Part model, mm, in its own coordinate system. Face numbers are marked on the shaded views. A direction names the side the tool comes from. Coordinates: 2 decimals unless noted, no trailing zeros. Order: outer loops, then holes, each group sorted by start corner. A loop starts at its lowest first (then second) coordinate and runs counter-clockwise, first axis right, second up.
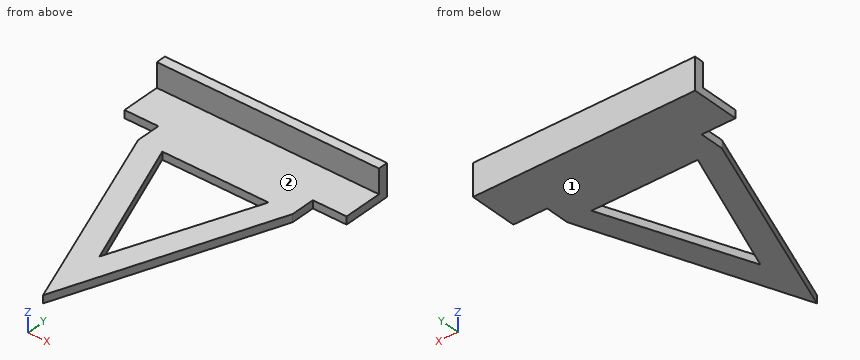
from build123d import *

# Parameters (mm, degrees)
F1_DEPTH = 1.6
F2_W     = 46
F2_H     = 2
F3_DEPTH = 5


with BuildPart() as f1:
    # F0 (on Top) → F1 (new body)
    with BuildSketch(Plane.XY):
        Polygon((23, 0), (0, 0), (-23, 0), (-23, -10), (-16, -10), (-16, -15), (0, -57.71), (16, -15), (16, -10), (23, -10), align=None)
        Polygon((0, -43.71), (-11, -15), (0, -15), (11, -15), align=None, mode=Mode.SUBTRACT)
    extrude(amount=F1_DEPTH)

    # F2 (on face) → F3 (join)
    with BuildSketch(Plane.XY.offset(1.6)):
        with Locations((0, -1)):
            Rectangle(F2_W, F2_H)
    extrude(amount=F3_DEPTH)


solid = f1.part
Q1. Cut at A-A on z = 0.75. Write the cut outline in (x, y).
Results list:
outline: (-23, -10) - (-16, -10) - (-16, -15) - (0, -57.71) - (16, -15) - (16, -10) - (23, -10) - (23, 0) - (-23, 0) - close; hole (-11, -15) - (0, -43.71) - (11, -15) - close
Q2. Pin check, flat tips, straight feed: pin 1 Ø1.3 at (y, z) = (-12.5, 1) entering from -X; pin 2 Ø6 at (x, y) = (-18, -22) entering from +Z; pin 3 Ø0.8 at (x, z) = (21, 1) entering from -Y; pin 4 Ø1.5 at (x, z) = (2, 4) entering from -Y. Stop position of each tip, or through.
Results list:
pin 1: stops at x = -16
pin 2: passes through
pin 3: stops at y = -10
pin 4: stops at y = -2
Q3. Wall check: line 1 along X through (y, z) = (-14.5, 1); line 2 along Y through (x, z) = (-17.5, 1); line 3 along Z through (x, y) = (-12, -17.5). Give the ranges that are in metal, low to high.
Results list:
line 1: x = -16 to 16
line 2: y = -10 to 0
line 3: z = 0 to 1.6
Q4. Which spindle directions (+Z, -Z, +X, -X, +Y, -Y) get a long thin tool onto all of the face, cutting with end or side? Do the marked faces 1 and 2. Say none if no direction does.
Results list:
face 1: -Z, +X, -X, +Y, -Y
face 2: +Z, +X, -X, -Y
Q5. Cut at C-C on y = -35.5. Write the cut outline in (x, z).
Results list:
outline: (-8.32, 0) - (-3.15, 0) - (-3.15, 1.6) - (-8.32, 1.6) - close; (3.15, 0) - (8.32, 0) - (8.32, 1.6) - (3.15, 1.6) - close
Q6. Cut at B-B on x = 10. Write the cut outline in (y, z).
Results list:
outline: (-31.02, 0) - (-17.61, 0) - (-17.61, 1.6) - (-31.02, 1.6) - close; (-15, 0) - (0, 0) - (0, 6.6) - (-2, 6.6) - (-2, 1.6) - (-15, 1.6) - close
Q7. Cut at D-D on x = 4.5. Write the cut outline in (y, z) (3 decimals).
Results list:
outline: (-45.698, 0) - (-31.965, 0) - (-31.965, 1.6) - (-45.698, 1.6) - close; (-15, 0) - (0, 0) - (0, 6.6) - (-2, 6.6) - (-2, 1.6) - (-15, 1.6) - close
